Could you check a few things on this model? Use its own coordinates, in mm. A direction names the side the tool comes from. Round coordinates to 2 decimals unless told otherwise and drop trailing zeros. Loops run counter-clockwise (first coordinate to the right, second up) from the corner with the lowest first, then second, coordinate; pieces in that order, holes last. Notation, with made-up numbers: (64, 65) -> (68, 65) arc R17 cw to (68, 80) -> close; hole circle Ø1 at (57.25, -25.75). An arc over 180 degrees is marked (long way). One line per item, written item: value.
```python
from build123d import *

# Parameters (mm, degrees)
SKETCH2_W           = 1500
SKETCH2_H           = 2198.57
BOSS_EXTRUDE1_DEPTH = 10
SKETCH3_W           = 480
SKETCH3_H           = 698.5704
SKETCH3_W_2         = 460
CUT_EXTRUDE1_DEPTH  = 1746.724604551
CUT_EXTRUDE3_DEPTH  = 10
CUT_EXTRUDE4_DEPTH  = 1746.724604551
BOSS_EXTRUDE2_DEPTH = 3
BOSS_EXTRUDE3_DEPTH = 3
SKETCH13_R          = 5
CUT_EXTRUDE5_DEPTH  = 1829.189928544
SKETCH14_R          = 5
CUT_EXTRUDE6_DEPTH  = 1829.189928544
SKETCH15_W          = 66
SKETCH15_H          = 26
BOSS_EXTRUDE5_DEPTH = 10
SKETCH16_W          = 66
SKETCH16_H          = 26
BOSS_EXTRUDE9_DEPTH = 10


with BuildPart() as part:
    # Sketch2 → Boss-Extrude1 (new body)
    with BuildSketch(Plane.XY):
        with Locations((79.505300353, -436.740830389)):
            Rectangle(SKETCH2_W, SKETCH2_H)
    extrude(amount=BOSS_EXTRUDE1_DEPTH)

    # Sketch3 → Cut-Extrude1 (cut, through all)
    with BuildSketch(Plane.XY.offset(10)):
        with Locations((79.505300353, 313.258969611)):
            Rectangle(SKETCH3_W, SKETCH3_H)
        with Locations((-440.494699647, 313.258969611)):
            Rectangle(SKETCH3_W_2, SKETCH3_H)
        with Locations((599.505300353, 313.258969611)):
            Rectangle(SKETCH3_W_2, SKETCH3_H)
    extrude(amount=-CUT_EXTRUDE1_DEPTH, mode=Mode.SUBTRACT)

    # Sketch9 → Cut-Extrude3 (cut)
    with BuildSketch(Plane(origin=(0, 0, 0), x_dir=(-1, 0, 0), z_dir=(0, 0, -1))):
        Polygon((-369.505300353, -36.026230389), (-829.505300353, -36.026230389), (-829.505300353, -1536.025830389), align=None)
        Polygon((210.494699647, -36.026230389), (670.494699647, -1536.025830389), (670.494699647, -36.026230389), align=None)
    extrude(amount=-CUT_EXTRUDE3_DEPTH, mode=Mode.SUBTRACT)

    # Sketch10 → Cut-Extrude4 (cut, through all)
    with BuildSketch(Plane(origin=(0, 0, 0), x_dir=(-1, 0, 0), z_dir=(0, 0, -1))):
        Polygon((-319.505300353, -86.026230389), (-779.505300353, -1536.025830389), (620.494699647, -1536.025830389), (160.494699647, -86.026230389), align=None)
    extrude(amount=-CUT_EXTRUDE4_DEPTH, mode=Mode.SUBTRACT)

    # Sketch11 → Boss-Extrude2 (add)
    with BuildSketch(Plane.ZY.offset(-319.505300353)):
        Polygon((0, 662.544169611), (42.246296146, 689.288336489), (52.943962897, 672.389818031), (-23.099370165, 624.250317651), (-33.797036917, 641.148836109), align=None)
    extrude(amount=-BOSS_EXTRUDE2_DEPTH)

    # Sketch12 → Boss-Extrude3 (add)
    with BuildSketch(Plane(origin=(-160.494699647, 0, 0), x_dir=(0, 0, -1), z_dir=(1, 0, 0))):
        Polygon((0, 662.544169611), (33.797036917, 641.148836109), (23.099370165, 624.250317651), (-52.943962897, 672.389818031), (-42.246296146, 689.288336489), align=None)
    extrude(amount=-BOSS_EXTRUDE3_DEPTH)

    # Sketch13 → Cut-Extrude5 (cut, through all)
    with BuildSketch(Plane(origin=(-160.494699647, 0, 0), x_dir=(0, 0, -1), z_dir=(1, 0, 0))):
        with Locations(Location((-34.683917705, 672.665589051, 0), (0, 0, 90))):
            Circle(SKETCH13_R)
        with Locations(Location((12.037265881, 643.088578886, 0), (0, 0, 90))):
            Circle(SKETCH13_R)
    extrude(amount=-CUT_EXTRUDE5_DEPTH, mode=Mode.SUBTRACT)

    # Sketch14 → Cut-Extrude6 (cut, through all)
    with BuildSketch(Plane.ZY.offset(-319.505300353)):
        with Locations(Location((32.895909771, 671.533684318, 0), (0, 0, 270))):
            Circle(SKETCH14_R)
        with Locations(Location((-16.256513993, 640.412580131, 0), (0, 0, 270))):
            Circle(SKETCH14_R)
    extrude(amount=-CUT_EXTRUDE6_DEPTH, mode=Mode.SUBTRACT)

    # Sketch15 → Boss-Extrude5 (add)
    with BuildSketch(Plane.XZ.offset(1536.025830389)):
        with Locations((804.505300353, 5)):
            Rectangle(SKETCH15_W, SKETCH15_H)
    extrude(amount=-BOSS_EXTRUDE5_DEPTH)

    # Sketch16 → Boss-Extrude9 (add)
    with BuildSketch(Plane.XZ.offset(1536.025830389)):
        with Locations((-645.494699647, 5)):
            Rectangle(SKETCH16_W, SKETCH16_H)
    extrude(amount=-BOSS_EXTRUDE9_DEPTH)


solid = part.part
```
Item 1: If we section it at C-C on x = 244: List the corners of the cut face in (y, z) for me, plus the area to 3 significant figures.
Output:
outline: (-86.03, 0) -> (-36.03, 0) -> (-36.03, 10) -> (-86.03, 10) -> close
area: 500 mm²
Item 2: If we section it at A-A on y = -296: List the corners of the cut face in (x, z) for me.
Output:
outline: (-290.22, 0) -> (-227.11, 0) -> (-227.11, 10) -> (-290.22, 10) -> close; (386.12, 0) -> (449.23, 0) -> (449.23, 10) -> (386.12, 10) -> close
Item 3: If we mould it in two halves opening along X, with no side actions, what happens to faces 3 (the face through (319.505, 355, 7)), 4 (the face through (-163.495, 668, 26)), 5 (the face through (601.17, -791.46, 4.93))? For each: released by +X, released by -X, zero draft, split by the parting line, or undercut.
Output:
face 3: undercut
face 4: released by -X
face 5: released by +X
Item 4: I need wall thicknesses on line 1 (X direction, y = 431, z = 4); line 2 (Z direction, x = -444.5, y = -835); line 3 (X direction, y = -718.5, z = 6.5). Which ranges of each line are inside material? Lowest first, please. Write a range as from..to.
Output:
line 1: x = -210.49..-160.49, 319.51..369.51
line 2: z = 0..10
line 3: x = -419.79..-361.14, 520.15..578.8
Item 5: Will these pins go through, and if not, where does the flat tip stop? pin 1 Ø6 at (y, z) = (671.53, 32.9) entering from -X; pin 2 Ø12 at (x, z) = (-45, 8) entering from +Y; pin 3 Ø11 at (x, z) = (-194.5, 4.5) entering from +Y.
Output:
pin 1: stops at x = -163.49
pin 2: stops at y = -36.03
pin 3: stops at y = 662.54
Item 6: If we section it at D-D on x = -411: List the corners of the cut face in (y, z) for me, plus the area to 3 significant figures.
Output:
outline: (-875.66, 0) -> (-689.85, 0) -> (-689.85, 10) -> (-875.66, 10) -> close
area: 1,860 mm²
Item 7: If we section it at B-B on y = -818: List the corners of the cut face in (x, z) for me, plus the area to 3 significant figures.
Output:
outline: (-450.3, 0) -> (-392.71, 0) -> (-392.71, 10) -> (-450.3, 10) -> close; (551.72, 0) -> (609.31, 0) -> (609.31, 10) -> (551.72, 10) -> close
area: 1,150 mm²
Item 8: For faces 1 (the face through (-435.763, -770.596, 4.93)), 2 (the face through (-160.495, 355, 6)), which set-ups out of +Z, -Z, +X, -X, +Y, -Y let a thin tool reach every point of the face, with its end or its side?
Output:
face 1: +Z, -Z, -X, +Y
face 2: +Z, -Z, +Y
